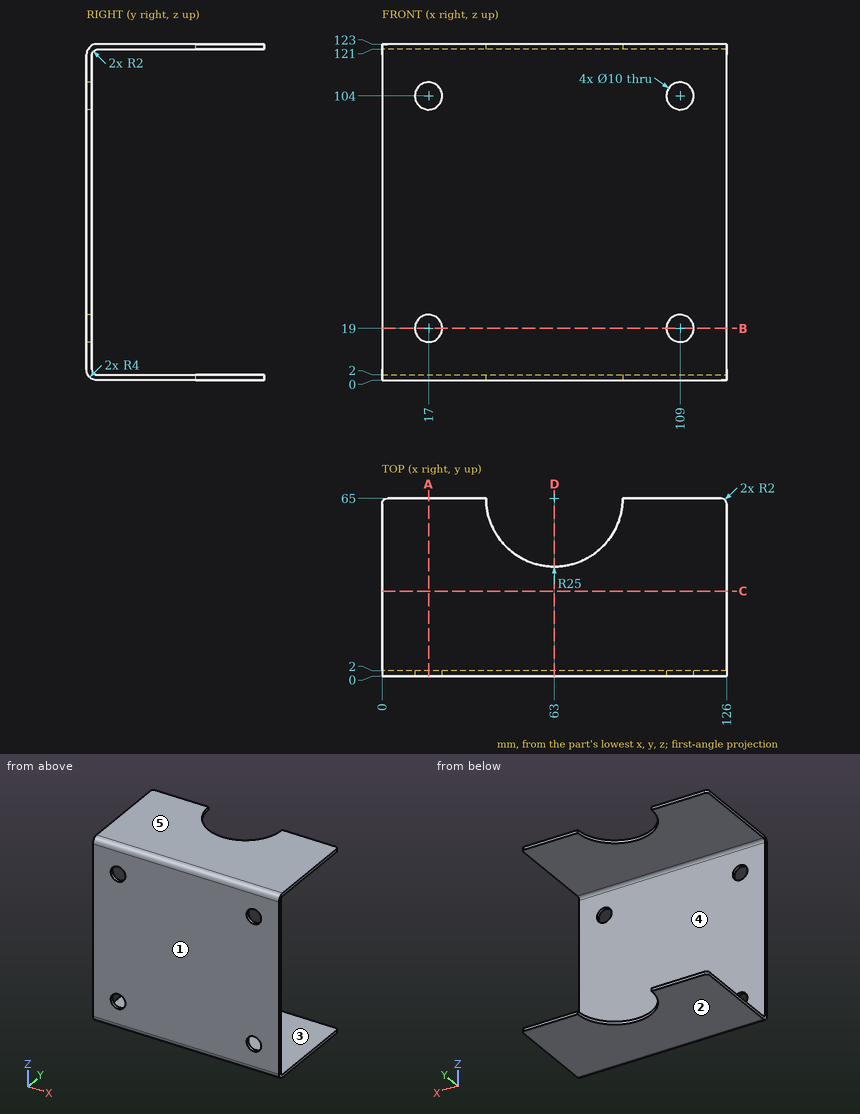
Can you work these out from the drawing? Everything is in mm from the part's minimum corner. A direction names the side the tool comes from. Round coordinates to 2 decimals unless told otherwise and drop trailing zeros. Loops run counter-clockwise (first coordinate to the right, second up) from the corner with the lowest first, then second, coordinate; pieces in that order, holes last. Notation, with made-up numbers: (-10, -34) - (26, -34) arc R17 ccw to (26, -18) - close; hole circle Ø3 at (-33, 82). An arc over 180 degrees is marked (long way). Answer in a Markdown table with one row per item. Add a question column.
(1) If we mould it in two halves opening along Z, with no side actions, what happens to the marked faces 1, 2 and 3? For each: pulls with the +Z half, pulls with the -Z half, needs draft (parallel to the pull), parting line crosses it, or undercut.
(2) For the marked faces 4 and 5, which set-ups out of +Z, -Z, +X, -X, +Y, -Y let a thin tool reach every point of the face, with its end or its side?
(3) If we section it at C-C (y = 31): Please give me the cut outline in (x, z).
(4) I'm going to push flat-ended pins straight in: pin 1 (16 mm diameter, centred on x = 109, z = 104, fed in from -Y); pin 2 (8 mm diameter, centred on x = 17, z = 19, fed in from +Y); pin 3 (11.5 mm diameter, centred on x = 17, z = 104, fed in from +Y). Where does each tip first touch, or does it pass through?
(5) If we section it at D-D (x = 63): Please give me the cut outline in (y, z).
(6) I need wall thicknesses on line 1 along Z through (x, y) = (102.5, 56); line 2 along Y through (x, z) = (28, 107); line 3 along Z through (x, y) = (109, 1.5). Which ranges of each line are inside material? Lowest first, please.
(7) If we section it at B-B (z = 19): Please give me the cut outline in (x, y).
(8) If we section it at A-A (x = 17): Please give me the cut outline in (y, z), plus the area to 3 significant figures.
Model answer:
| question | item | result |
|---|---|---|
| 1 | face 1 | needs draft |
| 1 | face 2 | pulls with the -Z half |
| 1 | face 3 | undercut |
| 2 | face 4 | +X, -X, +Y |
| 2 | face 5 | +Z, +X, -X, +Y, -Y |
| 3 | outline | (0, 0) - (126, 0) - (126, 2) - (0, 2) - close; (0, 121) - (126, 121) - (126, 123) - (0, 123) - close |
| 4 | pin 1 | stops at y = 0 |
| 4 | pin 2 | passes through |
| 4 | pin 3 | stops at y = 2 |
| 5 | outline | (0, 4) arc R4 ccw to (4, 0) - (40, 0) - (40, 2) - (4, 2) arc R2 cw to (2, 4) - (2, 119) arc R2 cw to (4, 121) - (40, 121) - (40, 123) - (4, 123) arc R4 ccw to (0, 119) - close |
| 6 | line 1 | z = 0 to 2, 121 to 123 |
| 6 | line 2 | y = 0 to 2 |
| 6 | line 3 | z = 0.88 to 14, 24 to 99, 109 to 122.12 |
| 7 | outline | (0, 0) - (12, 0) - (12, 2) - (0, 2) - close; (22, 0) - (104, 0) - (104, 2) - (22, 2) - close; (114, 0) - (126, 0) - (126, 2) - (114, 2) - close |
| 8 | outline | (0, 4) arc R4 ccw to (4, 0) - (65, 0) - (65, 2) - (4, 2) arc R2 cw to (2, 4) - (2, 14) - (0, 14) - close; (0, 24) - (2, 24) - (2, 99) - (0, 99) - close; (0, 109) - (2, 109) - (2, 119) arc R2 cw to (4, 121) - (65, 121) - (65, 123) - (4, 123) arc R4 ccw to (0, 119) - close |
| 8 | area | 453 mm² |
